Could you check a few things on this model? Use its own coordinates, in mm. Give positions to 0.01 mm unless a question says otherwise; leave off trailing zeros. Order: outer loops, then holes, each group sorted by start corner. A loop starts at its lowest first (then second) coordinate and runs counter-clockwise, first axis right, second up. Notation, with made-up numbers: (0.25, 48.5) - (25.25, 48.5) arc R12 cw to (25.25, 67.5) - close; hole circle Ø9 at (48, 45). An arc over 180 degrees is marked (long way). Put each result on its own line as item: value.
from build123d import *

# Parameters (mm, degrees)
BOSS_EXTRUDE1_DEPTH = 3.175
SCALE2_SCALE        = 0.962039453
SKETCH2_W           = 6.35
SKETCH2_H           = 3.175
BOSS_EXTRUDE2_DEPTH = 3.175


with BuildPart() as part:
    # Sketch1 → Boss-Extrude1 (new body)
    with BuildSketch(Plane.XY):
        with BuildLine():
            Line((-147.158374537, -62.773274702), (169.668548728, -62.773274702))
            ThreePointArc((169.668548728, -62.773274702), (11.255087096, 5.432872204), (-147.158374537, -62.773274702))
        make_face()
        with BuildLine():
            Line((50.41023946, -57.693274702), (94.019934732, -57.693274702))
            ThreePointArc((94.019934732, -57.693274702), (96.211786347, -56.436780252), (96.235095135, -53.910429423))
            Line((96.235095135, -53.910429423), (74.430247499, -15.046995704))
            ThreePointArc((74.430247499, -15.046995704), (72.215087096, -13.749840983), (69.999926692, -15.046995704))
            Line((69.999926692, -15.046995704), (48.195079056, -53.910429423))
            ThreePointArc((48.195079056, -53.910429423), (48.218387844, -56.436780252), (50.41023946, -57.693274702))
        make_face(mode=Mode.SUBTRACT)
        with BuildLine():
            Line((105.763734274, -54.380906597), (126.29666869, -37.319025838))
            ThreePointArc((126.29666869, -37.319025838), (127.208455368, -35.207887623), (126.042260143, -33.225906744))
            ThreePointArc((126.042260143, -33.225906744), (105.546270909, -21.656125731), (83.898857508, -12.418436605))
            ThreePointArc((83.898857508, -12.418436605), (81.096030012, -13.162488886), (80.817372324, -16.048975619))
            Line((80.817372324, -16.048975619), (101.925252726, -53.670183739))
            ThreePointArc((101.925252726, -53.670183739), (103.677973758, -54.924887225), (105.763734274, -54.380906597))
        make_face(mode=Mode.SUBTRACT)
        with BuildLine():
            Line((44.287940881, -50.492254775), (66.833764967, -10.308156511))
            ThreePointArc((66.833764967, -10.308156511), (66.956550428, -8.072532741), (65.262680667, -6.608328129))
            ThreePointArc((65.262680667, -6.608328129), (42.578611895, -1.963069006), (19.524331112, 0.19228386))
            ThreePointArc((19.524331112, 0.19228386), (17.300963083, -0.95402892), (17.138389089, -3.450219634))
            Line((17.138389089, -3.450219634), (39.785454632, -50.353828112))
            ThreePointArc((39.785454632, -50.353828112), (41.994726342, -51.788209913), (44.287940881, -50.492254775))
        make_face(mode=Mode.SUBTRACT)
        with BuildLine():
            Line((-21.777766689, -50.492254775), (-44.323590776, -10.308156511))
            ThreePointArc((-44.323590776, -10.308156511), (-44.446376237, -8.072532741), (-42.752506476, -6.608328129))
            ThreePointArc((-42.752506476, -6.608328129), (-20.068437704, -1.963069006), (2.985843079, 0.19228386))
            ThreePointArc((2.985843079, 0.19228386), (5.209211108, -0.95402892), (5.371785102, -3.450219634))
            Line((5.371785102, -3.450219634), (-17.275280441, -50.353828112))
            ThreePointArc((-17.275280441, -50.353828112), (-19.484552151, -51.788209913), (-21.777766689, -50.492254775))
        make_face(mode=Mode.SUBTRACT)
        with BuildLine():
            Line((-58.307198133, -16.048975619), (-79.415078535, -53.670183739))
            ThreePointArc((-79.415078535, -53.670183739), (-81.167799567, -54.924887225), (-83.253560083, -54.380906597))
            Line((-83.253560083, -54.380906597), (-103.786494499, -37.319025838))
            ThreePointArc((-103.786494499, -37.319025838), (-104.698281177, -35.207887623), (-103.532085952, -33.225906744))
            ThreePointArc((-103.532085952, -33.225906744), (-83.036096718, -21.656125731), (-61.388683317, -12.418436605))
            ThreePointArc((-61.388683317, -12.418436605), (-58.585855821, -13.162488886), (-58.307198133, -16.048975619))
        make_face(mode=Mode.SUBTRACT)
        with BuildLine():
            Line((-128.343015855, -57.693274702), (-94.247026375, -57.693274702))
            ThreePointArc((-94.247026375, -57.693274702), (-91.858128819, -56.016274393), (-92.623705231, -53.199706566))
            Line((-92.623705231, -53.199706566), (-109.306769117, -39.336883017))
            ThreePointArc((-109.306769117, -39.336883017), (-110.836303138, -38.752183245), (-112.404816005, -39.222412473))
            ThreePointArc((-112.404816005, -39.222412473), (-121.401975006, -46.004337694), (-130.027908578, -53.252554703))
            ThreePointArc((-130.027908578, -53.252554703), (-130.717824142, -56.054321649), (-128.343015855, -57.693274702))
        make_face(mode=Mode.SUBTRACT)
        with BuildLine():
            Line((13.542412941, -7.685960278), (35.928399311, -54.048856086))
            ThreePointArc((35.928399311, -54.048856086), (35.792447827, -56.503529625), (33.641073466, -57.693274702))
            Line((33.641073466, -57.693274702), (-11.130899275, -57.693274702))
            ThreePointArc((-11.130899275, -57.693274702), (-13.282273636, -56.503529625), (-13.41822512, -54.048856086))
            Line((-13.41822512, -54.048856086), (8.96776125, -7.685960278))
            ThreePointArc((8.96776125, -7.685960278), (11.255087096, -6.250378893), (13.542412941, -7.685960278))
        make_face(mode=Mode.SUBTRACT)
        with BuildLine():
            Line((-25.684904865, -53.910429423), (-47.489752501, -15.046995704))
            ThreePointArc((-47.489752501, -15.046995704), (-49.704912904, -13.749840983), (-51.920073308, -15.046995704))
            Line((-51.920073308, -15.046995704), (-73.724920944, -53.910429423))
            ThreePointArc((-73.724920944, -53.910429423), (-73.701612156, -56.436780252), (-71.50976054, -57.693274702))
            Line((-71.50976054, -57.693274702), (-27.900065268, -57.693274702))
            ThreePointArc((-27.900065268, -57.693274702), (-25.708213653, -56.436780252), (-25.684904865, -53.910429423))
        make_face(mode=Mode.SUBTRACT)
        with BuildLine():
            Line((115.133879422, -53.199706566), (131.816943308, -39.336883017))
            ThreePointArc((131.816943308, -39.336883017), (133.346477329, -38.752183245), (134.914990196, -39.222412473))
            ThreePointArc((134.914990196, -39.222412473), (143.912149197, -46.004337694), (152.538082769, -53.252554703))
            ThreePointArc((152.538082769, -53.252554703), (153.227998333, -56.054321649), (150.853190046, -57.693274702))
            Line((150.853190046, -57.693274702), (116.757200566, -57.693274702))
            ThreePointArc((116.757200566, -57.693274702), (114.36830301, -56.016274393), (115.133879422, -53.199706566))
        make_face(mode=Mode.SUBTRACT)
    extrude(amount=BOSS_EXTRUDE1_DEPTH)


with BuildPart() as part_1:
    # Scale2: scaled about (11.255087096, -36.675334956, 1.5875)
    add(part.part.scale(SCALE2_SCALE).moved(Location((0.427249265, -1.392215783, 0.060262369))))

    # Sketch2 → Boss-Extrude2 (add)
    with BuildSketch(Plane.XY.offset(3.114737631)):
        with Locations((-103.044912854, -63.370082629)):
            Rectangle(SKETCH2_W, SKETCH2_H)
        with Locations((-64.944912854, -63.370082629)):
            Rectangle(SKETCH2_W, SKETCH2_H)
        with Locations((-26.844912854, -63.370082629)):
            Rectangle(SKETCH2_W, SKETCH2_H)
        with Locations((11.255087146, -63.370082629)):
            Rectangle(SKETCH2_W, SKETCH2_H)
        with Locations((49.355087146, -63.370082629)):
            Rectangle(SKETCH2_W, SKETCH2_H)
        with Locations((87.455087146, -63.370082629)):
            Rectangle(SKETCH2_W, SKETCH2_H)
        with Locations((125.555087146, -63.370082629)):
            Rectangle(SKETCH2_W, SKETCH2_H)
    extrude(amount=-BOSS_EXTRUDE2_DEPTH)


solid = part_1.part
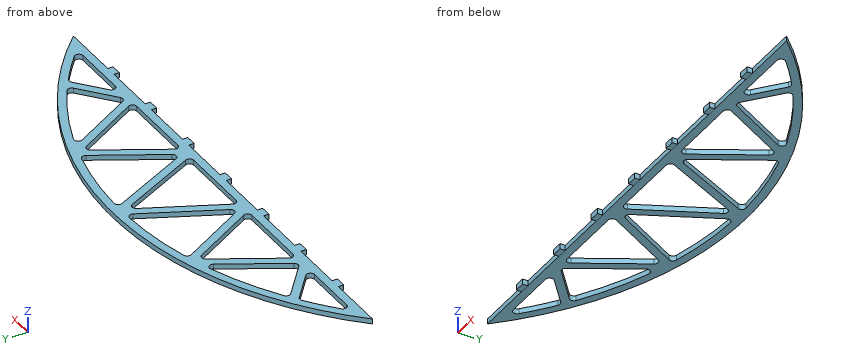
1) Suppose I cut it at A-A, the plane x = -94. List the corners of the cut face in (y, z) for me, and give its area (3 significant figures).
Filled in:
outline: (-61.78, 0.06) - (-56.9, 0.06) - (-56.9, 3.11) - (-61.78, 3.11) - close; (-48.15, 0.06) - (-41.8, 0.06) - (-41.8, 3.11) - (-48.15, 3.11) - close; (-30.15, 0.06) - (-24.48, 0.06) - (-24.48, 3.11) - (-30.15, 3.11) - close
area: 51.7 mm^2
2) Suppose I cut it at D-D, the plane x = -3.5. List the corners of the cut face in (y, z) for me, and give its area (3 significant figures).
Filled in:
outline: (-61.78, 0.06) - (-56.9, 0.06) - (-56.9, 3.11) - (-61.78, 3.11) - close; (-34.79, 0.06) - (-23.55, 0.06) - (-23.55, 3.11) - (-34.79, 3.11) - close; (-1.58, 0.06) - (3.31, 0.06) - (3.31, 3.11) - (-1.58, 3.11) - close
area: 64.2 mm^2
3) Suppose I cut it at B-B, the plane y = -22.5. State how many separate pieces and enclosed holes the cut face has, and give its area (3 significant figures).
Filled in:
separate pieces: 8
enclosed holes: 0
area: 166 mm^2
4) I'm going to push flat-ended pins straight in: pin 1 (1.6 mm diameter, centred on y = -63.5, z = 1.5, fed in from -X); pin 2 (1.5 mm diameter, centred on x = 2, z = 1.5, fed in from +Y); pin 3 (1 mm diameter, centred on y = -37.5, z = 1, fed in from -X). Where does each tip first touch, or does it pass through?
Filled in:
pin 1: stops at x = -106.22
pin 2: stops at y = 3.66
pin 3: stops at x = -114.45
5) If I drill on line 1 (Y direction, x = -31, z = 0.1); line 2 (Y direction, x = 90, z = 1.9) (3 decimals); line 3 (X direction, y = -11.5, z = 1.9), over which ranges is the centre line in solid material (lowest first)? Write a range as [from, to].
Filled in:
line 1: y = [-61.78, -56.9], [-41.28, -31.3], [-5.46, -0.47]
line 2: y = [-64.958, -56.895], [-47.893, -37.905], [-16.788, -11.505]
line 3: x = [-67.48, -42.11], [2.32, 7.74], [14.77, 20.19], [64.62, 89.99]
